```python
from build123d import *

# Parameters (mm, degrees)
F0_R     = 35
F0_R_2   = 3
F0_R_3   = 4
F1_DEPTH = 8
F2_R     = 5
F2_R_2   = 4
F3_DEPTH = 7
F6_D     = 3.4


with BuildPart() as f1:
    # F0 (on Top) → F1 (new body)
    with BuildSketch(Plane.XY):
        Circle(F0_R)
        with Locations((-15, -25.9807621135)):
            Circle(F0_R_2, mode=Mode.SUBTRACT)
        with Locations((-25.9807621135, -15)):
            Circle(F0_R_2, mode=Mode.SUBTRACT)
        with BuildLine():
            ThreePointArc((-14.1520683747, -20.6087107971), (-20.2390786896, -14.6758200382), (-23.9864227741, -7.0463836473))
            ThreePointArc((-23.9864227741, -7.0463836473), (-23.7500595541, -4.779622232), (-21.9889424597, -3.3330602854))
            Line((-21.9889424597, -3.3330602854), (-11.4594190982, -1.7370064413))
            ThreePointArc((-11.4594190982, -1.7370064413), (-5.7054148294, -4.143495838), (-5.1972611447, -10.3597275079))
            Line((-5.1972611447, -10.3597275079), (-9.8028524215, -19.5400764091))
            ThreePointArc((-9.8028524215, -19.5400764091), (-11.7379895363, -21.049011774), (-14.1520683747, -20.6087107971))
        make_face(mode=Mode.SUBTRACT)
        with Locations((0, -30)):
            Circle(F0_R_2, mode=Mode.SUBTRACT)
        with Locations((15, -25.9807621135)):
            Circle(F0_R_2, mode=Mode.SUBTRACT)
        with BuildLine():
            ThreePointArc((21.9889424597, -3.3330602854), (23.7500595541, -4.779622232), (23.9864227741, -7.0463836473))
            ThreePointArc((23.9864227741, -7.0463836473), (20.2390786896, -14.6758200382), (14.1520683747, -20.6087107971))
            ThreePointArc((14.1520683747, -20.6087107971), (11.7379895363, -21.049011774), (9.8028524215, -19.5400764091))
            Line((9.8028524215, -19.5400764091), (5.1972611447, -10.3597275079))
            ThreePointArc((5.1972611447, -10.3597275079), (5.7054148294, -4.143495838), (11.4594190982, -1.7370064413))
            Line((11.4594190982, -1.7370064413), (21.9889424597, -3.3330602854))
        make_face(mode=Mode.SUBTRACT)
        with Locations((25.9807621135, -15)):
            Circle(F0_R_2, mode=Mode.SUBTRACT)
        with Locations((-30, 0)):
            Circle(F0_R_2, mode=Mode.SUBTRACT)
        with Locations((-25.9807621135, 15)):
            Circle(F0_R_2, mode=Mode.SUBTRACT)
        with BuildLine():
            ThreePointArc((-23.9864227741, 7.0463836473), (-20.2390786896, 14.6758200382), (-14.1520683747, 20.6087107971))
            ThreePointArc((-14.1520683747, 20.6087107971), (-11.7379895363, 21.049011774), (-9.8028524215, 19.5400764091))
            Line((-9.8028524215, 19.5400764091), (-5.1972611447, 10.3597275079))
            ThreePointArc((-5.1972611447, 10.3597275079), (-5.7054148294, 4.143495838), (-11.4594190982, 1.7370064413))
            Line((-11.4594190982, 1.7370064413), (-21.9889424597, 3.3330602854))
            ThreePointArc((-21.9889424597, 3.3330602854), (-23.7500595541, 4.779622232), (-23.9864227741, 7.0463836473))
        make_face(mode=Mode.SUBTRACT)
        with Locations((-15, 25.9807621135)):
            Circle(F0_R_2, mode=Mode.SUBTRACT)
        Circle(F0_R_3, mode=Mode.SUBTRACT)
        with BuildLine():
            ThreePointArc((9.8028524215, 19.5400764091), (11.7379895363, 21.049011774), (14.1520683747, 20.6087107971))
            ThreePointArc((14.1520683747, 20.6087107971), (20.2390786896, 14.6758200382), (23.9864227741, 7.0463836473))
            ThreePointArc((23.9864227741, 7.0463836473), (23.7500595541, 4.779622232), (21.9889424597, 3.3330602854))
            Line((21.9889424597, 3.3330602854), (11.4594190982, 1.7370064413))
            ThreePointArc((11.4594190982, 1.7370064413), (5.7054148294, 4.143495838), (5.1972611447, 10.3597275079))
            Line((5.1972611447, 10.3597275079), (9.8028524215, 19.5400764091))
        make_face(mode=Mode.SUBTRACT)
        with Locations((30, 0)):
            Circle(F0_R_2, mode=Mode.SUBTRACT)
        with Locations((25.9807621135, 15)):
            Circle(F0_R_2, mode=Mode.SUBTRACT)
        with Locations((15, 25.9807621135)):
            Circle(F0_R_2, mode=Mode.SUBTRACT)
        with Locations((0, 30)):
            Circle(F0_R_2, mode=Mode.SUBTRACT)
    extrude(amount=F1_DEPTH)

    # F2 (on face) → F3 (join)
    with BuildSketch(Plane.XY.offset(8)):
        Circle(F2_R)
        Circle(F2_R_2, mode=Mode.SUBTRACT)
    extrude(amount=F3_DEPTH)

    # F6 (through all)
    with Locations(Plane.XZ.offset(5)):
        with Locations((0, 11)):
            Hole(F6_D / 2)


solid = f1.part
```
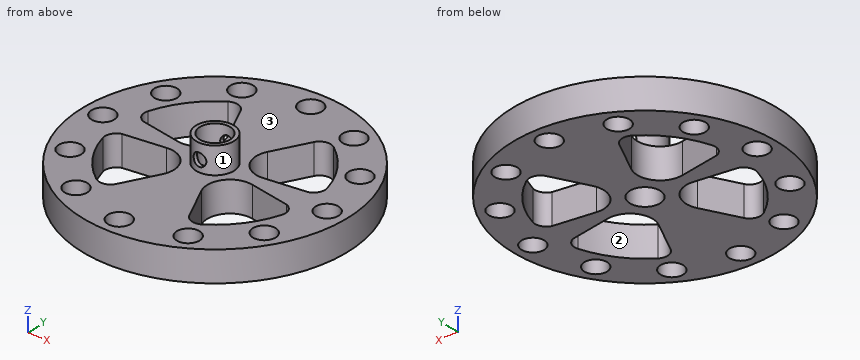
Input: part model. Units: mm. Frame: model coordinates. Face numbers are marked on the shaded views. Give positions to 0.01 mm unless a question says otherwise; leave off trailing zeros. Order: outer loops, then holes, each group sorted by start corner. A loop starts at its lowest first (then second) coordinate and runs counter-clockwise, first axis right, second up. Notation, with made-up numbers: (-13.75, 87.5) -> (45.25, 87.5) arc R32 ccw to (45.25, 123.5) -> close; hole circle Ø6 at (-34.75, -31). An arc over 180 degrees is marked (long way). Write each question's results on one line, items separated by ' | '. Start each with the question number.
Item 1: Cut plane C-C on y = -30. Return the cut outline in (x, z).
Item 2: Cut plane D-D on x = -15. Return the cut outline in (y, z), then the cut area to 3 significant figures.
Item 3: Cut plane A-A on x = 0. Return the cut outline in (y, z).
Item 4: Line query: line 1 (Y direction, x = 15, z = 6); line 2 (Y direction, x = -20, z = 7); line 3 (X direction, y = -16, z = 4). Output: solid intervals per line, ascending.
Item 5: Mould query, pull axis Y, two halves, no side actions, for the marked faces 1, 2 and 3. Classes: pulls with the +Y half, pulls with the -Y half, needs draft (parallel to the pull), parting line crosses it, or undercut.
Item 6: Cut plane B-B on y = 0. Return the cut outline in (x, z).
Item 7: Contact query for flat-ended pins moving along their axis: P1, Ø1.5, axis at x = -27, y = 21, coming from the +Z side; P2, Ø2, axis at y = -16.5, z = 5.5, coming from the +X side; P3, Ø10.5, axis at x = 0, y = 0, coming from the +Z side; P4, Ø3.5, axis at x = 25.98, y = -15, coming from the +Z side. Output: stop coordinate, or through.
Established:
1) outline: (-18.03, 0) -> (-3, 0) -> (-3, 8) -> (-18.03, 8) -> close; (3, 0) -> (18.03, 0) -> (18.03, 8) -> (3, 8) -> close
2) outline: (-31.62, 0) -> (-28.98, 0) -> (-28.98, 8) -> (-31.62, 8) -> close; (-22.98, 0) -> (-20, 0) -> (-20, 8) -> (-22.98, 8) -> close; (-2.27, 0) -> (2.27, 0) -> (2.27, 8) -> (-2.27, 8) -> close; (20, 0) -> (22.98, 0) -> (22.98, 8) -> (20, 8) -> close; (28.98, 0) -> (31.62, 0) -> (31.62, 8) -> (28.98, 8) -> close | area: 126 mm^2
3) outline: (-35, 0) -> (-33, 0) -> (-33, 8) -> (-35, 8) -> close; (-27, 0) -> (-4, 0) -> (-4, 9.3) -> (-5, 9.3) -> (-5, 8) -> (-27, 8) -> close; (-5, 12.7) -> (-4, 12.7) -> (-4, 15) -> (-5, 15) -> close; (4, 0) -> (27, 0) -> (27, 8) -> (5, 8) -> (5, 9.3) -> (4, 9.3) -> close; (4, 12.7) -> (5, 12.7) -> (5, 15) -> (4, 15) -> close; (33, 0) -> (35, 0) -> (35, 8) -> (33, 8) -> close
4) line 1: -31.62 to -28.98, -22.98 to -20, -2.27 to 2.27, 20 to 22.98, 28.98 to 31.62 | line 2: -28.72 to -15, -3.03 to 3.03, 15 to 28.72 | line 3: -31.13 to -28.81, -23.15 to -19.21, -8.03 to 8.03, 19.21 to 23.15, 28.81 to 31.13
5) face 1: parting line crosses it | face 2: undercut | face 3: needs draft
6) outline: (-35, 0) -> (-33, 0) -> (-33, 8) -> (-35, 8) -> close; (-27, 0) -> (-4, 0) -> (-4, 15) -> (-5, 15) -> (-5, 8) -> (-27, 8) -> close; (4, 0) -> (27, 0) -> (27, 8) -> (5, 8) -> (5, 15) -> (4, 15) -> close; (33, 0) -> (35, 0) -> (35, 8) -> (33, 8) -> close
7) P1: z = 8 | P2: x = 31.38 | P3: z = 15 | P4: through
